from build123d import *

# Parameters (mm, degrees)
SKETCH1_W           = 54.61
SKETCH1_H           = 39.6875
BOSS_EXTRUDE1_DEPTH = 21.0185
CHAMFER1_SIZE       = 8.261835623
SKETCH2_R           = 19.05
BOSS_EXTRUDE2_DEPTH = 73.025
SKETCH3_R           = 6.35
BOSS_EXTRUDE3_DEPTH = 2.54
BOSS_EXTRUDE4_DEPTH = 196.85
BOSS_EXTRUDE5_DEPTH = 11.43
SKETCH6_R           = 10.00125
CUT_EXTRUDE1_DEPTH  = 203.2
SKETCH7_W           = 17.653
SKETCH7_H           = 8.8265
BOSS_EXTRUDE6_DEPTH = 19.1643
CHAMFER2_SIZE       = 3.81
CUT_EXTRUDE2_DEPTH  = 17.653
CHAMFER3_SIZE       = 0.889


with BuildPart() as part:
    # Sketch1 → Boss-Extrude1 (new body)
    with BuildSketch(Plane(origin=(0, 0, 0), x_dir=(0, 0, -1), z_dir=(1, 0, 0))):
        with Locations((27.305, 19.84375)):
            Rectangle(SKETCH1_W, SKETCH1_H)
        with BuildLine():
            ThreePointArc((54.61, 39.6875), (74.45375, 19.84375), (54.61, 0))
            Line((54.61, 0), (54.61, 39.6875))
        make_face()
    extrude(amount=BOSS_EXTRUDE1_DEPTH)

    # Chamfer1
    chamfer1_edges = [part.edges().sort_by_distance(p)[0] for p in [
        (10.50925, 0, 0),
        (10.50925, 39.6875, 0),
    ]]
    chamfer(chamfer1_edges, length=CHAMFER1_SIZE)

    # Sketch2 → Boss-Extrude2 (add)
    with BuildSketch(Plane.ZY):
        with Locations((-54.61, 19.84375)):
            Circle(SKETCH2_R)
    extrude(amount=BOSS_EXTRUDE2_DEPTH)

    # Sketch3 → Boss-Extrude3 (add)
    with BuildSketch(Plane.ZY.offset(73.025)):
        with Locations((-54.61, 19.84375)):
            Circle(SKETCH3_R)
    extrude(amount=BOSS_EXTRUDE3_DEPTH)

    # Sketch4 → Boss-Extrude4 (add)
    with BuildSketch(Plane.ZY):
        with BuildLine():
            ThreePointArc((-14.7066, 5.13715), (-4.307463412, 9.444613412), (0, 19.84375))
            Line((0, 19.84375), (-14.7066, 19.84375))
            Line((-14.7066, 19.84375), (-34.925, 19.84375))
            Line((-34.925, 19.84375), (-34.925, 9.906))
            Line((-34.925, 9.906), (-14.7066, 5.13715))
        make_face()
        with BuildLine():
            Line((-14.7066, 19.84375), (0, 19.84375))
            ThreePointArc((0, 19.84375), (-4.307463412, 30.242886588), (-14.7066, 34.55035))
            Line((-14.7066, 34.55035), (-34.925, 29.7815))
            Line((-34.925, 29.7815), (-34.925, 19.84375))
            Line((-34.925, 19.84375), (-14.7066, 19.84375))
        make_face()
    extrude(amount=BOSS_EXTRUDE4_DEPTH)

    # Sketch5 → Boss-Extrude5 (add)
    with BuildSketch(Plane.ZY.offset(196.85)):
        with BuildLine():
            Line((-34.925, 19.84375), (0, 19.84375))
            ThreePointArc((0, 19.84375), (-4.307463412, 30.242886588), (-14.7066, 34.55035))
            Line((-14.7066, 34.55035), (-34.925, 29.7815))
            Line((-34.925, 29.7815), (-34.925, 19.84375))
        make_face()
        with BuildLine():
            Line((0, 19.84375), (1.168107566, 19.84375))
            ThreePointArc((1.168107566, 19.84375), (-3.481486631, 31.068863369), (-14.7066, 35.718457566))
            Line((-14.7066, 35.718457566), (-35.852392434, 30.7975))
            Line((-35.852392434, 30.7975), (-35.852392434, 19.84375))
            Line((-35.852392434, 19.84375), (-34.925, 19.84375))
            Line((-34.925, 19.84375), (-34.925, 29.7815))
            Line((-34.925, 29.7815), (-14.7066, 34.55035))
            ThreePointArc((-14.7066, 34.55035), (-4.307463412, 30.242886588), (0, 19.84375))
        make_face()
        with BuildLine():
            ThreePointArc((-14.7066, 5.13715), (-4.307463412, 9.444613412), (0, 19.84375))
            Line((0, 19.84375), (-34.925, 19.84375))
            Line((-34.925, 19.84375), (-34.925, 9.906))
            Line((-34.925, 9.906), (-14.7066, 5.13715))
        make_face()
        with BuildLine():
            ThreePointArc((-14.7066, 3.969042434), (-3.481486631, 8.618636631), (1.168107566, 19.84375))
            Line((1.168107566, 19.84375), (0, 19.84375))
            ThreePointArc((0, 19.84375), (-4.307463412, 9.444613412), (-14.7066, 5.13715))
            Line((-14.7066, 5.13715), (-34.925, 9.906))
            Line((-34.925, 9.906), (-34.925, 19.84375))
            Line((-34.925, 19.84375), (-35.852392434, 19.84375))
            Line((-35.852392434, 19.84375), (-35.852392434, 8.89))
            Line((-35.852392434, 8.89), (-14.7066, 3.969042434))
        make_face()
    extrude(amount=BOSS_EXTRUDE5_DEPTH)

    # Sketch6 → Cut-Extrude1 (cut)
    with BuildSketch(Plane.ZY.offset(208.28)):
        with Locations((-14.7066, 19.84375)):
            Circle(SKETCH6_R)
    extrude(amount=-CUT_EXTRUDE1_DEPTH, mode=Mode.SUBTRACT)

    # Sketch7 → Boss-Extrude6 (add)
    with BuildSketch(Plane(origin=(21.0185, 0, 0), x_dir=(0, 0, -1), z_dir=(1, 0, 0))):
        with Locations((19.6215, 15.4305)):
            Rectangle(SKETCH7_W, SKETCH7_H)
        with Locations((19.6215, 24.257)):
            Rectangle(SKETCH7_W, SKETCH7_H)
    extrude(amount=BOSS_EXTRUDE6_DEPTH)

    # Chamfer2
    chamfer2_edges = [part.edges().sort_by_distance(p)[0] for p in [
        (30.60065, 11.01725, -10.795),
        (30.60065, 11.01725, -28.448),
        (30.60065, 28.67025, -28.448),
        (30.60065, 28.67025, -10.795),
    ]]
    chamfer(chamfer2_edges, length=CHAMFER2_SIZE)

    # Sketch8 → Cut-Extrude2 (cut)
    with BuildSketch(Plane.XZ.offset(-11.01725)):
        with BuildLine():
            ThreePointArc((28.6385, -19.6215), (31.7119, -22.6949), (34.7853, -19.6215))
            Line((34.7853, -19.6215), (28.6385, -19.6215))
        make_face()
        with BuildLine():
            Line((28.6385, -19.6215), (34.7853, -19.6215))
            ThreePointArc((34.7853, -19.6215), (31.7119, -16.5481), (28.6385, -19.6215))
        make_face()
    extrude(amount=-CUT_EXTRUDE2_DEPTH, mode=Mode.SUBTRACT)

    # Chamfer3
    chamfer3_edges = [part.edges().sort_by_distance(p)[0] for p in [
        (40.1828, 19.84375, -10.795),
        (40.1828, 28.67025, -19.6215),
        (40.1828, 11.01725, -19.6215),
        (40.1828, 19.84375, -28.448),
        (40.1828, 12.92225, -12.7),
        (40.1828, 12.92225, -26.543),
        (40.1828, 26.76525, -26.543),
        (40.1828, 26.76525, -12.7),
    ]]
    chamfer(chamfer3_edges, length=CHAMFER3_SIZE)


solid = part.part
Input: part model. Units: mm. Frame: model coordinates. A direction names the side the tool comes from. Round coordinates to 2 decimals unless told otherwise and drop trailing zeros. Order: outer loops, then holes, each group sorted by start corner. A loop starts at its lowest first (then second) coordinate and runs counter-clockwise, first axis right, second up.
1. Material intervals for line 1 (Z direction, x = -60, y = 14) (3 decimals); line 2 (X direction, y = 28, z = -35); line 3 (X direction, y = 16, z = -47) (1 decimal), sorted ascending.
The answers:
line 1: z = -72.742 to -36.478, -34.925 to -22.823, -6.59 to -1.211
line 2: x = -208.28 to -196.85, 0 to 21.02
line 3: x = -73 to 21
2. Cut plane C-C, the plane x = -114.5. Output: boundary loops of the cut face in (y, z) (1 decimal).
The answers:
outline: (5.1, -14.7) - (9.9, -34.9) - (29.8, -34.9) - (34.6, -14.7) arc R14.7 ccw to start; hole circle Ø20 at (19.8, -14.7)
3. Cut plane A-A, the plane x = -55.5. State how many separate pieces and enclosed holes the cut face has, then the cut area to 3 significant figures.
The answers:
separate pieces: 2
enclosed holes: 1
area: 1,660 mm2
4. Cut plane D-D, the plane z = -40. Output: boundary loops of the cut face in (x, y) (1 decimal), then the cut area to 3 significant figures.
The answers:
outline: (-73, 7.6) - (0, 7.6) - (0, 0) - (21, 0) - (21, 39.7) - (0, 39.7) - (0, 32.1) - (-73, 32.1) - close
area: 2,620 mm2
5. Set-up query: faces 1 (the face through (-74.28, 15.98, -59.65)), 2 (the face through (-97.05, 32.2, -24.67)), 3 (the face through (-97, 20, -34.925)), 4 (the face through (-196.85, 33, -23)). Return all of +Z, -Z, +X, -X, +Y, -Y with unobstructed straight access to the full face (end or side cutting, diameter ignored); none if empty.
The answers:
face 1: -X
face 2: +Y
face 3: +Y, -Y
face 4: none
6. Cut plane B-B, the plane x = 25. Output: boundary loops of the cut face in (y, z) (3 decimals), then the cut area to 3 significant figures.
The answers:
outline: (11.017, -24.638) - (14.827, -28.448) - (24.86, -28.448) - (28.67, -24.638) - (28.67, -14.605) - (24.86, -10.795) - (14.827, -10.795) - (11.017, -14.605) - close
area: 283 mm2
7. Pin query (flat end, axial travel): P1, Ø8, axis at x = 29.5, y = 18.5, coming from the +Z side (3 decimals); P2, Ø11, axis at x = 34, z = -18.5, coming from the +Y side; P3, Ø3, axis at x = -68.5, z = -44.5, coming from the +Y side; P4, Ø3.5, axis at x = 31.71, z = -19.62, coming from the +Y side. Return the tip coordinate at first contact, or that it passes through.
The answers:
P1: stops at z = -10.795
P2: stops at y = 28.67
P3: stops at y = 36.84
P4: passes through
8. Mould query, pull axis Y, two halves, no side actions, for faces 5 (the face through (-108.1, 29.76, -16.01)), 6 (the face through (-202, 20, -35.852)), 7 (the face through (39.74, 13.21, -26.2)), 8 (the face through (-5.08, 20, -15)). Classes: released by +Y, released by -Y, zero draft, split by the parting line, or undercut.
The answers:
face 5: undercut
face 6: zero draft
face 7: released by -Y
face 8: undercut
